from build123d import *

# Parameters (mm, degrees)
CROQUIS1_W              = 25
CROQUIS1_H              = 20
SALIENTE_EXTRUIR1_DEPTH = 21.7
CROQUIS2_W              = 2.5
CROQUIS2_H              = 20
SALIENTE_EXTRUIR2_DEPTH = 43.5
CROQUIS3_W              = 25
CROQUIS3_H              = 20
SALIENTE_EXTRUIR3_DEPTH = 2.5
CROQUIS4_R              = 2.25
CORTAR_EXTRUIR1_DEPTH   = 10
CROQUIS6_R              = 2
CORTAR_EXTRUIR2_DEPTH   = 10
CORTAR_EXTRUIR4_DEPTH   = 70
SALIENTE_EXTRUIR5_DEPTH = 15
CORTAR_EXTRUIR5_DEPTH   = 15
CORTAR_EXTRUIR6_DEPTH   = 20
CORTAR_EXTRUIR7_START   = -65.2
CORTAR_EXTRUIR7_DEPTH   = 65.2


with BuildPart() as part:
    # Croquis1 → Saliente-Extruir1 (new body)
    with BuildSketch(Plane.XY):
        with Locations((12.5, 10)):
            Rectangle(CROQUIS1_W, CROQUIS1_H)
    extrude(amount=SALIENTE_EXTRUIR1_DEPTH)

    # Croquis2 → Saliente-Extruir2 (add)
    with BuildSketch(Plane.XY.offset(21.7)):
        with Locations((1.25, 10)):
            Rectangle(CROQUIS2_W, CROQUIS2_H)
        with Locations((23.75, 10)):
            Rectangle(CROQUIS2_W, CROQUIS2_H)
    extrude(amount=SALIENTE_EXTRUIR2_DEPTH)

    # Croquis3 → Saliente-Extruir3 (add)
    with BuildSketch(Plane.XY.offset(65.2)):
        with Locations((12.5, 10)):
            Rectangle(CROQUIS3_W, CROQUIS3_H)
    extrude(amount=-SALIENTE_EXTRUIR3_DEPTH)

    # Croquis4 → Cortar-Extruir1 (cut)
    with BuildSketch(Plane.XZ):
        with Locations(Location((7, 18.2, 0), (0, 0, 270))):
            Circle(CROQUIS4_R)
        with Locations(Location((18, 18.2, 0), (0, 0, 270))):
            Circle(CROQUIS4_R)
    extrude(amount=-CORTAR_EXTRUIR1_DEPTH, mode=Mode.SUBTRACT)

    # Croquis6 → Cortar-Extruir2 (cut)
    with BuildSketch(Plane(origin=(0, 0, 0), x_dir=(-1, 0, 0), z_dir=(0, 0, -1))):
        with Locations((-2.5, 5)):
            Circle(CROQUIS6_R)
        with Locations((-22.5, 5)):
            Circle(CROQUIS6_R)
    extrude(amount=-CORTAR_EXTRUIR2_DEPTH, mode=Mode.SUBTRACT)

    # Croquis10 → Cortar-Extruir4 (cut)
    with BuildSketch(Plane(origin=(25, 0, 0), x_dir=(0, 0, -1), z_dir=(1, 0, 0))):
        Polygon((-65.2, 0), (-24.1, 0), (-65.2, 15), align=None)
    extrude(amount=-CORTAR_EXTRUIR4_DEPTH, mode=Mode.SUBTRACT)

    # Croquis11 → Saliente-Extruir5 (add)
    with BuildSketch(Plane(origin=(0, 0, 0), x_dir=(-1, 0, 0), z_dir=(0, 0, -1))):
        Polygon((-25, 1.920937271), (-30.856516071, -2.764275585), (-28.982430928, -5.106882014), (-23.125914857, -0.421669157), (-21.632203551, 0.773299888), align=None)
    saliente_extruir5 = extrude(amount=-SALIENTE_EXTRUIR5_DEPTH)

    # Croquis12 → Cortar-Extruir5 (cut)
    with BuildSketch(Plane(origin=(8.81905499, 11.023818737, 0), x_dir=(0.7808688094430302, -0.6246950475544245, 0), z_dir=(-0.6246950475544245, -0.7808688094430302, 0))):
        Polygon((19.521720236, 15), (25.821720236, 0), (25.821720236, 15), align=None)
    cortar_extruir5 = extrude(amount=-CORTAR_EXTRUIR5_DEPTH, mode=Mode.SUBTRACT)

    # Simetría1: Saliente-Extruir5, Cortar-Extruir5 across plane
    add(saliente_extruir5.mirror(Plane(origin=(12.5, 0, 0), x_dir=(0, 0, 1), z_dir=(1, 0, 0))))
    add(cortar_extruir5.mirror(Plane(origin=(12.5, 0, 0), x_dir=(0, 0, 1), z_dir=(1, 0, 0))), mode=Mode.SUBTRACT)

    # Croquis13 → Cortar-Extruir6 (cut)
    with BuildSketch(Plane.XZ):
        with BuildLine():
            Line((9.5, -11.99123488), (9.5, 11.99123488))
            ThreePointArc((9.5, 11.99123488), (12.5, 14.99123488), (15.5, 11.99123488))
            Line((15.5, 11.99123488), (15.5, -11.99123488))
            ThreePointArc((15.5, -11.99123488), (12.5, -14.99123488), (9.5, -11.99123488))
        make_face()
    extrude(amount=-CORTAR_EXTRUIR6_DEPTH, mode=Mode.SUBTRACT)

    # Croquis14 → Cortar-Extruir7 (cut)
    with BuildSketch(Plane(origin=(0, 0, 0), x_dir=(-1, 0, 0), z_dir=(0, 0, -1)).offset(CORTAR_EXTRUIR7_START)):
        with BuildLine():
            Line((-25, 10.960468636), (-27.59046433, 24.120971106))
            Line((-27.59046433, 24.120971106), (2.993644675, 24.120971106))
            Line((2.993644675, 24.120971106), (0, 10.960468636))
            ThreePointArc((0, 10.960468636), (-12.5, 23.460468636), (-25, 10.960468636))
        make_face()
    extrude(amount=CORTAR_EXTRUIR7_DEPTH, mode=Mode.SUBTRACT)


solid = part.part
Work out the finished part from the listing and answer in its coordinate system (mm). A direction names the side the tool comes from. Give positions to 0.01 mm unless a question says otherwise; leave off trailing zeros. Loops run counter-clockwise (first coordinate to the right, second up) from the corner with the lowest first, then second, coordinate; pieces in that order, holes last. Notation, with made-up numbers: (-33, 49.25) -> (-8, 49.25) arc R31 ccw to (-8, 84.25) -> close; hole circle Ø6 at (-4, 24). An arc over 180 degrees is marked (long way). Use a Markdown table: item, result. Add a question column.
1) Consider line 1 along X through (y, z) = (7, 18.2); line 2 along Z through (x, y) = (6, 18); line 3 along X through (y, z) = (11.5, 5). Determine where each line is inside the solid, lowest interval first.
2) The part is cut by section B-B, the plane z = 55.5. Determine the outline of the cut face in (x, y), plus the area to 3 significant figures.
3) The part is cut by section D-D, the plane z = 18.5. Determine the outline of the cut face in (x, y), plus the area to 3 significant figures.
4) Each of these flat-tipped pins is pushed along its axis until it touches: P1, Ø15, axis at y = 8, z = 36, coming from the -X side; P2, Ø6, axis at x = 10.5, z = 15.5, coming from the -Y side; P3, Ø2, axis at x = 3, y = 4.5, coming from the -Z side. Where does it stop, or does it pass through?
5) The part is cut by section A-A, the plane x = 12.5. Determine the outline of the cut face in (y, z), plus the area to 3 significant figures.
6) The part is cut by section C-C, the plane x = 18. Determine the outline of the cut face in (y, z), plus the area to 3 significant figures.
7) For a pull along Y with two mould halves and no side action, classify faces 5 (the flat face through (18, 10, 18)), 6 (the cylindrical face through (24.498, 5.088, 4.93)), 7 (the flat face through (12, 20, 64)), 8 (the cylindrical face through (8.52, 4.93, 19.86)) as +Y half, -Y half, draft (parallel to the pull), parting line (faces both ways), or undercut.
8) Which of the six approach directions +Z, -Z, +X, -X, +Y, -Y give full straight-line access (tool end or side, diameter ignored) to faces 1 (the flat face through (9.5, 10, 6)), 2 (the flat face through (15, 0, 15)), 3 (the flat face through (2.5, 11, 37)), 4 (the flat face through (3, 5, 10))?
Reported:
| question | item | result |
|---|---|---|
| 1 | line 1 | x = 0 to 4.75, 9.25 to 15.75, 20.25 to 25 |
| 1 | line 2 | z = 0 to 21.7, 62.7 to 65.2 |
| 1 | line 3 | x = 0.01 to 9.5, 15.5 to 24.99 |
| 2 | outline | (0.01, 11.46) -> (2.5, 11.46) -> (2.5, 18.46) arc R12.5 ccw to start; (22.5, 11.46) -> (24.99, 11.46) arc R12.5 ccw to (22.5, 18.46) -> close |
| 2 | area | 23.1 mm^2 |
| 3 | outline | (0, 0) -> (4.77, 0) -> (4.77, 10) -> (9.23, 10) -> (9.23, 0) -> (15.77, 0) -> (15.77, 10) -> (20.23, 10) -> (20.23, 0) -> (25, 0) -> (25, 10.96) arc R12.5 ccw to (21.13, 20) -> (3.87, 20) arc R12.5 ccw to (0, 10.96) -> close |
| 3 | area | 389 mm^2 |
| 4 | P1 | stops at x = 0 |
| 4 | P2 | stops at y = 0 |
| 4 | P3 | stops at z = 10 |
| 5 | outline | (0, 14.99) -> (20, 14.99) -> (20, 21.7) -> (0, 21.7) -> close; (14.09, 62.7) -> (20, 62.7) -> (20, 65.2) -> (15, 65.2) -> close |
| 5 | area | 148 mm^2 |
| 6 | outline | (0, 0) -> (20, 0) -> (20, 21.7) -> (0, 21.7) -> (0, 20.45) -> (10, 20.45) -> (10, 15.95) -> (0, 15.95) -> close; (14.09, 62.7) -> (20, 62.7) -> (20, 65.2) -> (15, 65.2) -> close |
| 6 | area | 403 mm^2 |
| 7 | face 5 | -Y half |
| 7 | face 6 | undercut |
| 7 | face 7 | +Y half |
| 7 | face 8 | draft |
| 8 | face 1 | -Z, +Y, -Y |
| 8 | face 2 | +Z, -Y |
| 8 | face 3 | +Y, -Y |
| 8 | face 4 | -Z |
